```python
from build123d import *

# Parameters (mm, degrees)
MODEL_R             = 0.4445
MODEL_R_2           = 0.3
BOSS_EXTRUDE1_DEPTH = 1.65
SKETCH2_W           = 2.85
SKETCH2_H           = 6.858
BOSS_EXTRUDE2_DEPTH = 3.5
SKETCH3_W           = 1.5
SKETCH3_H           = 3
BOSS_EXTRUDE3_DEPTH = 0.66
SKETCH4_W           = 1.25
SKETCH4_H           = 2
BOSS_EXTRUDE4_DEPTH = 1.4
SKETCH5_W           = 2
SKETCH5_H           = 5.1
BOSS_EXTRUDE5_DEPTH = 1.17
SKETCH6_W           = 8.61
SKETCH6_H           = 2.92
BOSS_EXTRUDE6_DEPTH = 1.62
SKETCH7_W           = 9.63
SKETCH7_H           = 4.32
BOSS_EXTRUDE7_DEPTH = 2.17
SKETCH8_W           = 3
SKETCH8_H           = 4
BOSS_EXTRUDE8_DEPTH = 1.5
SKETCH9_R           = 1
BOSS_EXTRUDE9_DEPTH = 0.5


with BuildPart() as part:
    # Model → Boss-Extrude1 (new body)
    with BuildSketch(Plane.XY):
        with BuildLine():
            Line((3, 35.5), (32, 35.5))
            ThreePointArc((32, 35.5), (34.121320344, 34.621320344), (35, 32.5))
            Line((35, 32.5), (35, 32.2))
            Line((35, 32.2), (36, 32.2))
            Line((36, 32.2), (36, 23.2))
            Line((36, 23.2), (35, 23.2))
            Line((35, 23.2), (35, 12))
            Line((35, 12), (36, 12))
            Line((36, 12), (36, 3))
            Line((36, 3), (35, 3))
            ThreePointArc((35, 3), (34.121320344, 0.878679656), (32, 0))
            Line((32, 0), (22, 0))
            Line((22, 0), (22, 0.5))
            Line((22, 0.5), (11.1, 0.5))
            Line((11.1, 0.5), (11.1, 0))
            Line((11.1, 0), (3, 0))
            ThreePointArc((3, 0), (0.878679656, 0.878679656), (0, 3))
            Line((0, 3), (0, 32.5))
            ThreePointArc((0, 32.5), (0.878679656, 34.621320344), (3, 35.5))
        make_face()
        with Locations((7.8, 2.54)):
            Circle(MODEL_R, mode=Mode.SUBTRACT)
        with Locations((2.72, 1.524)):
            Circle(MODEL_R, mode=Mode.SUBTRACT)
        with Locations((2.72, 3.556)):
            Circle(MODEL_R, mode=Mode.SUBTRACT)
        with Locations((17, 32.3)):
            Circle(MODEL_R_2, mode=Mode.SUBTRACT)
        with Locations((23.54, 32.3)):
            Circle(MODEL_R_2, mode=Mode.SUBTRACT)
        with Locations((30.76, 25.494)):
            Circle(MODEL_R_2, mode=Mode.SUBTRACT)
    extrude(amount=BOSS_EXTRUDE1_DEPTH)

    # Sketch2 → Boss-Extrude2 (add)
    with BuildSketch(Plane.XY.offset(1.65)):
        with Locations((34.275, 27.7)):
            Rectangle(SKETCH2_W, SKETCH2_H)
        with Locations((34.275, 7.5)):
            Rectangle(SKETCH2_W, SKETCH2_H)
    extrude(amount=BOSS_EXTRUDE2_DEPTH)

    # Sketch3 → Boss-Extrude3 (add)
    with BuildSketch(Plane(origin=(35.7, 0, 0), x_dir=(0, 0, -1), z_dir=(1, 0, 0))):
        with Locations((-3.4, 27.7)):
            Rectangle(SKETCH3_W, SKETCH3_H)
        with Locations((-3.4, 7.5)):
            Rectangle(SKETCH3_W, SKETCH3_H)
    extrude(amount=BOSS_EXTRUDE3_DEPTH)

    # Sketch4 → Boss-Extrude4 (add)
    with BuildSketch(Plane.XY.offset(1.65)):
        with Locations((1.855, 8.16)):
            Rectangle(SKETCH4_W, SKETCH4_H)
    extrude(amount=BOSS_EXTRUDE4_DEPTH)

    # Sketch5 → Boss-Extrude5 (add)
    with BuildSketch(Plane.XY.offset(1.65)):
        with Locations((2.2, 29.73)):
            Rectangle(SKETCH5_W, SKETCH5_H)
    extrude(amount=BOSS_EXTRUDE5_DEPTH)

    # Sketch6 → Boss-Extrude6 (add)
    with BuildSketch(Plane.XY.offset(1.65)):
        with Locations((20.105, 31.9)):
            Rectangle(SKETCH6_W, SKETCH6_H)
    extrude(amount=BOSS_EXTRUDE6_DEPTH)

    # Sketch7 → Boss-Extrude7 (add)
    with BuildSketch(Plane.XY.offset(1.65)):
        with Locations((16.815, 3.77)):
            Rectangle(SKETCH7_W, SKETCH7_H)
    extrude(amount=BOSS_EXTRUDE7_DEPTH)

    # Sketch8 → Boss-Extrude8 (add)
    with BuildSketch(Plane.XY.offset(1.65)):
        with Locations((8.8, 16.47)):
            Rectangle(SKETCH8_W, SKETCH8_H)
    extrude(amount=BOSS_EXTRUDE8_DEPTH)

    # Sketch9 → Boss-Extrude9 (add)
    with BuildSketch(Plane.XY.offset(3.15)):
        with Locations((8.8, 16.47)):
            Circle(SKETCH9_R)
    extrude(amount=BOSS_EXTRUDE9_DEPTH)


solid = part.part
```
Part model, mm, in its own coordinate system. A direction names the side the tool comes from. Round coordinates to 2 decimals unless told otherwise and drop trailing zeros. Order: outer loops, then holes, each group sorted by start corner. A loop starts at its lowest first (then second) coordinate and runs counter-clockwise, first axis right, second up. Notation, with made-up numbers: M 7.25,88 L 43.25,88 A9 cw 43.25,102 Z; hole C 65.5,40 d3. An arc over 180 degrees is marked long. Answer in a Markdown table with one row per item. Add a question column.
Q1. 3-axis set-ups, long thin cutter, end or side, ignore diameter. For faces 1 (the face through (17, 5.93, 3)), 2 (the face through (34, 10.929, 3)), 3 (the face through (32.85, 7, 3)), 4 (the face through (35.5, 23.2, 0.8)): which of +Z, -Z, +X, -X, +Y, -Y reach the whole face in a straight line?
Q2. Cut at D-D on z = 0.45. Give the cut face in (x, y).
Q3. Wall check: L1, parallel to X at y = 32.3, z = 0.4; L2, parallel to Y at x = 30.76, z = 0.5; L3, parallel to Y at x = 33, z = 4.35. Give the ranges that are in metal, low to high. Write a range as from..to.
Q4. Cut at A-A on y = 2.54. Give the cut face in (x, z).
Q5. Mould opens along X. For faces 5 (the face through (34, 8, 5.15)), 6 (the face through (9.26, 15.58, 3.4)), 7 (the face through (17, 0.5, 1)) say: +X half, -X half, draft (parallel to the pull), parting line (faces both ways), or undercut.
Q6. Cut at B-B on x = 18. Give the cut face in (y, z), and give its area (3 significant figures).
Q7. Pin check, flat tips, straight feed: pin 1 (0.5 mm diameter, centred on x = 19, z = 3, fed in from -Y); pin 2 (1.5 mm diameter, centred on y = 19.5, z = 4, fed in from -X); pin 3 (2 mm diameter, centred on y = 7, z = 1, fed in from +X); pin 4 (1 mm diameter, centred on x = 2, z = 2.5, fed in from -Y). Stop position of each tip, or through.
Q8. Cut at C-C on y = 16.47. Give the cut face in (x, z).
Established:
| question | item | result |
|---|---|---|
| 1 | face 1 | +Z, -X |
| 1 | face 2 | +Z, +X, -X |
| 1 | face 3 | +Z, +Y, -Y |
| 1 | face 4 | +Z, -Z, +X |
| 2 | outline | M 0,3 A3 ccw 3,0 L 11.1,0 L 11.1,0.5 L 22,0.5 L 22,0 L 32,0 A3 ccw 35,3 L 36,3 L 36,12 L 35,12 L 35,23.2 L 36,23.2 L 36,32.2 L 35,32.2 L 35,32.5 A3 ccw 32,35.5 L 3,35.5 A3 ccw 0,32.5 Z; hole C 2.72,1.52 d0.89; hole C 2.72,3.56 d0.89; hole C 7.8,2.54 d0.89; hole C 17,32.3 d0.6; hole C 23.54,32.3 d0.6; hole C 30.76,25.49 d0.6 |
| 3 | L1 | x = 0..16.7, 17.3..23.24, 23.84..35 |
| 3 | L2 | y = 0..25.19, 25.79..35.5 |
| 3 | L3 | y = 4.07..10.93, 24.27..31.13 |
| 4 | outline | M 0.04,0 L 7.36,0 L 7.36,1.65 L 0.04,1.65 Z; M 8.24,0 L 34.96,0 L 34.96,1.65 L 21.63,1.65 L 21.63,3.82 L 12,3.82 L 12,1.65 L 8.24,1.65 Z |
| 5 | face 5 | draft |
| 5 | face 6 | parting line |
| 5 | face 7 | undercut |
| 6 | outline | M 0.5,0 L 35.5,0 L 35.5,1.65 L 33.36,1.65 L 33.36,3.27 L 30.44,3.27 L 30.44,1.65 L 5.93,1.65 L 5.93,3.82 L 1.61,3.82 L 1.61,1.65 L 0.5,1.65 Z |
| 6 | area | 71.9 mm2 |
| 7 | pin 1 | stops at y = 1.61 |
| 7 | pin 2 | passes through |
| 7 | pin 3 | stops at x = 36 |
| 7 | pin 4 | stops at y = 7.16 |
| 8 | outline | M 0,0 L 35,0 L 35,1.65 L 10.3,1.65 L 10.3,3.15 L 9.8,3.15 L 9.8,3.65 L 7.8,3.65 L 7.8,3.15 L 7.3,3.15 L 7.3,1.65 L 0,1.65 Z |
